from build123d import *

# Parameters (mm, degrees)
F0_W     = 50
F0_H     = 150
F1_DEPTH = 15
F2_R     = 5
F3_DEPTH = 25
F4_R     = 3
F5_DEPTH = 10
F6_R     = 3.1
F7_DEPTH = 10.2


with BuildPart() as f1:
    # F0 (on Top) → F1 (new body)
    with BuildSketch(Plane.XY):
        Rectangle(F0_W, F0_H)
    extrude(amount=F1_DEPTH)

    # F2 (on face) → F3 (cut)
    with BuildSketch(Plane.XY.offset(15)):
        with Locations((0, 40)):
            Circle(F2_R)
        Circle(F2_R)
        with Locations((0, -40)):
            Circle(F2_R)
    extrude(amount=-F3_DEPTH, mode=Mode.SUBTRACT)

    # F4 (on face) → F5 (join)
    with BuildSketch(Plane.YZ.offset(25)):
        with Locations((-40, 7.5)):
            Circle(F4_R)
        with Locations((0, 7.5)):
            Circle(F4_R)
        with Locations((40, 7.5)):
            Circle(F4_R)
    extrude(amount=F5_DEPTH)

    # F6 (on face) → F7 (cut)
    with BuildSketch(Plane(origin=(-25, 0, 0), x_dir=(0, -1, 0), z_dir=(-1, 0, 0))):
        with Locations((-40, 7.5)):
            Circle(F6_R)
        with Locations((0, 7.5)):
            Circle(F6_R)
        with Locations((40, 7.5)):
            Circle(F6_R)
    extrude(amount=-F7_DEPTH, mode=Mode.SUBTRACT)


solid = f1.part
Check sheet for the modelled part. Datum: model origin and axes. Units: mm. A direction names the side the tool comes from. Round coordinates to 2 decimals unless told otherwise and drop trailing zeros. Loops run counter-clockwise (first coordinate to the right, second up) from the corner with the lowest first, then second, coordinate; pieces in that order, holes last. Notation, with made-up numbers: (73, -12) -> (81, -12) arc R18 cw to (81, 6) -> close; hole circle Ø7 at (80.25, 61.5). An arc over 180 degrees is marked (long way). Put each result on its own line as item: value. Start each with the question number.
1. Gauge pin test, flat end, axial feed: pin 1 (1.9 mm diameter, centred on y = -41.5, z = 6.5, fed in from -X). Record the tip position at first contact, or that the pin passes through.
2. Section check A-A (x = 0). Enter the section's corners in (y, z).
3. Scan lines: probe 1 along Y at (x, z) = (0, 10.5); probe 2 along Z at (x, y) = (-17.5, -40); probe 3 along X at (y, z) = (-32, 8.75). Record each from-to range of solid material in increasing order.
4. Section check D-D (z = 7.5). Give the number of separate pieces and of enclosed holes in the cut face, plus the area to 3 significant figures.
5. Draft check along Z on faces 1 (the face through (29.9, -43, 7.6)), 2 (the face through (3, -36, 8)), 3 (the face through (-19.971, -42.864, 6.313)). Enter one of: +Z half, -Z half, draft (parallel to the pull), parting line (faces both ways), or undercut.
6. Section check C-C (z = 1.5). Enter the section's corners in (x, y).
7. Section check B-B (y = 0). Enter the section's corners in (x, z), plus the area to 3 significant figures.
8. Access from +Z, -Z, +X, -X, +Y, -Y to the whole of each face (thin tool, end or side, straight path). Record for faces 4 (the face through (-19.971, 0.404, 10.574)), 5 (the face through (0, -75, 7)), 6 (the face through (29.9, -3, 7.6)).
Findings:
1. pin 1: stops at x = -14.8
2. outline: (-75, 0) -> (-45, 0) -> (-45, 15) -> (-75, 15) -> close; (-35, 0) -> (-5, 0) -> (-5, 15) -> (-35, 15) -> close; (5, 0) -> (35, 0) -> (35, 15) -> (5, 15) -> close; (45, 0) -> (75, 0) -> (75, 15) -> (45, 15) -> close
3. probe 1: y = -75 to -45, -35 to -5, 5 to 35, 45 to 75
3. probe 2: z = 0 to 4.4, 10.6 to 15
3. probe 3: x = -25 to 25
4. separate pieces: 1
4. enclosed holes: 3
4. area: 7,250 mm^2
5. face 1: parting line
5. face 2: draft
5. face 3: undercut
6. outline: (-25, -75) -> (25, -75) -> (25, 75) -> (-25, 75) -> close; hole circle Ø10 at (0, -40); hole circle Ø10 at (0, 0); hole circle Ø10 at (0, 40)
7. outline: (-25, 0) -> (-5, 0) -> (-5, 15) -> (-25, 15) -> (-25, 10.6) -> (-14.8, 10.6) -> (-14.8, 4.4) -> (-25, 4.4) -> close; (5, 0) -> (25, 0) -> (25, 4.5) -> (35, 4.5) -> (35, 10.5) -> (25, 10.5) -> (25, 15) -> (5, 15) -> close
7. area: 597 mm^2
8. face 4: -X
8. face 5: +Z, -Z, +X, -X, -Y
8. face 6: +X
